from build123d import *

# Parameters (mm, degrees)
BOSS_EXTRUDE1_DEPTH = 5
BOSS_EXTRUDE2_START = 1.5
BOSS_EXTRUDE2_DEPTH = 1.5
FILLET1_R           = 1.5


with BuildPart() as part:
    # Sketch1 → Boss-Extrude1 (new body)
    with BuildSketch(Plane.XY):
        with BuildLine():
            Line((9.73, -20.13), (9.73, -24.18))
            ThreePointArc((9.73, -24.18), (7.48, -26.43), (5.23, -24.18))
            Line((5.23, -24.18), (5.23, -20.13))
            Line((5.23, -20.13), (5.14173141, -20.13))
            Line((5.14173141, -20.13), (2.80346282, -24.18))
            Line((2.80346282, -24.18), (5.14173141, -28.23))
            Line((5.14173141, -28.23), (9.81826859, -28.23))
            Line((9.81826859, -28.23), (12.15653718, -24.18))
            Line((12.15653718, -24.18), (9.81826859, -20.13))
            Line((9.81826859, -20.13), (9.73, -20.13))
        make_face()
    extrude(amount=-BOSS_EXTRUDE1_DEPTH)

    # Sketch2 → Boss-Extrude2 (add)
    with BuildSketch(Plane.XY.offset(BOSS_EXTRUDE2_START)):
        with BuildLine():
            Line((0.885, -17.25), (0.885, -19.25))
            Line((0.885, -19.25), (0.885, -24.18))
            ThreePointArc((0.885, -24.18), (7.48, -30.775), (14.075, -24.18))
            Line((14.075, -24.18), (14.075, -17.25))
            Line((14.075, -17.25), (10.575, -17.25))
            Line((10.575, -17.25), (9.73, -17.25))
            Line((9.73, -17.25), (9.73, -20.13))
            Line((9.73, -20.13), (9.73, -24.18))
            ThreePointArc((9.73, -24.18), (7.48, -26.43), (5.23, -24.18))
            Line((5.23, -24.18), (5.23, -20.13))
            Line((5.23, -20.13), (5.23, -17.25))
            Line((5.23, -17.25), (0.885, -17.25))
        make_face()
    extrude(amount=-BOSS_EXTRUDE2_DEPTH)

    # Fillet1
    fillet1_edges = [part.edges().sort_by_distance(p)[0] for p in [
        (9.73, -20.715, 1.5),
        (7.48, -26.43, 1.5),
        (5.23, -20.715, 1.5),
    ]]
    fillet(fillet1_edges, radius=FILLET1_R)


solid = part.part
The model under review builds one solid part; all positions refer to its coordinate system, in mm. A direction names the side the tool comes from. Give positions to 0.01 mm unless a question says otherwise; leave off trailing zeros. Order: outer loops, then holes, each group sorted by start corner. A loop starts at its lowest first (then second) coordinate and runs counter-clockwise, first axis right, second up. Notation, with made-up numbers: M 47,44.5 L 72,44.5 A38 cw 72,82.5 Z; hole C 73.25,23.25 d10. An arc over 180 degrees is marked long. Answer in a Markdown table with one row per item. Add a question column.
1. Add section B-B on x = 7.48. State the section outline as (y, z) points (3 decimals).
2. To check wall thickness, follow line 1 along Z through (x, y) = (11.75, -22); line 2 along X through (y, z) = (-21, 1.25) (3 decimals); line 3 along X through (y, z) = (-23, -2). State the ranges of each line that lie inside material, in increasing order.
3. For pin 1 Ø1.2 at (y, z) = (-21.5, -2.5) entering from +X; pin 2 Ø1.5 at (y, z) = (-28.5, -2) entering from -X; pin 3 Ø3 at (y, z) = (-25.5, -3) entering from -X, all flat-tipped, find the tip position at first contact; note any pin that passes through.
4. Add section D-D on x = 11.5. State the section outline as (y, z) points, plus the area to 3 significant figures.
5. Machinability: for faces 4 (the flat face through (11, -22.18, -2.46)), 5 (the flat face through (5.23, -22, -2)), 6 (the flat face through (4, -21, 0)), 7 (the flat face through (3.96, -26.18, -2.46)), which of the approach directions +Z, -Z, +X, -X, +Y, -Y give a long, thin tool a straight path to every point of the face, cutting with its end or side? Answer none if there is none.
6. Mouldability with a two-part tool opening along X and no side actions: class faces 1 (the flat face through (4, -27, 1.5)), 2 (the flat face through (10.971, -26.233, -2.465)), 3 (the cylindrical face through (4.8, -20.67, 1.05)) as released by +X, released by -X, zero draft, split by the parting line, or undercut.
7. Add section A-A on y = -18.25. State the section outline as (x, z) points (3 decimals), plus the area to 3 significant figures.
8. Add section C-C on z = -4. State the section outline as (x, y) points.
The answers:
| question | item | result |
|---|---|---|
| 1 | outline | M -30.775,0 L -28.23,0 L -28.23,-5 L -26.43,-5 L -26.43,0 A1.5 ccw -27.93,1.5 L -30.775,1.5 Z |
| 2 | line 1 | 0 to 1.5 |
| 2 | line 2 | 0.885 to 4.559, 10.401 to 14.075 |
| 2 | line 3 | 3.48 to 5.23, 9.73 to 11.48 |
| 3 | pin 1 | x = 10.96 |
| 3 | pin 2 | x = 4.86 |
| 3 | pin 3 | x = 2.8 |
| 4 | outline | M -29.41,0 L -25.32,0 L -25.32,-5 L -23.04,-5 L -23.04,0 L -17.25,0 L -17.25,1.5 L -29.41,1.5 Z |
| 4 | area | 29.6 mm2 |
| 5 | face 4 | -Z, +X, +Y |
| 5 | face 5 | +Z, -Z, +Y |
| 5 | face 6 | -Z |
| 5 | face 7 | -Z, -X, -Y |
| 6 | face 1 | zero draft |
| 6 | face 2 | released by +X |
| 6 | face 3 | undercut |
| 7 | outline | M 0.885,0 L 5.23,0 A1.5 ccw 3.73,1.5 L 0.885,1.5 Z; M 9.73,0 L 14.075,0 L 14.075,1.5 L 11.23,1.5 A1.5 ccw Z |
| 7 | area | 12.1 mm2 |
| 8 | outline | M 2.8,-24.18 L 5.14,-28.23 L 9.82,-28.23 L 12.16,-24.18 L 9.82,-20.13 L 9.73,-20.13 L 9.73,-24.18 A2.25 cw 5.23,-24.18 L 5.23,-20.13 L 5.14,-20.13 Z |
